Could you check a few things on this model? Use its own coordinates, in mm. A direction names the side the tool comes from. Round coordinates to 2 decimals unless told otherwise and drop trailing zeros. Loops run counter-clockwise (first coordinate to the right, second up) from the corner with the lowest first, then second, coordinate; pieces in that order, holes last. Notation, with made-up numbers: (-30, 3) -> (5, 3) arc R30 ccw to (5, 25) -> close; hole circle Ø11 at (9.5, 46.5). An arc over 180 degrees is marked (long way). Write each question's results on one line, items separated by ' | '. Start each with the question number.
1) Imagine slicing it at D-D, the plane z = -2.5. List the corners of the cut face in (x, y) for me.
2) Which directions (+Z, -Z, +X, -X, +Y, -Y) give clear straight access to the entire face, cutting with the end or side of a thin tool? Please do faces 4 (the flat face through (8.852, 21, 0)), 5 (the flat face through (4, 21.5, 2)), 6 (the flat face through (20, 8, 0)), 7 (the flat face through (-3, 15, 0)), 8 (the flat face through (-3, 15.8, 0)).
3) If I drill on probe 1 along Z at (x, y) = (21.5, 15.2); probe 2 along X at (y, z) = (9.25, -2.5); probe 3 along Y at (x, z) = (9.25, 0.5), over which ranges is the centre line in solid material (lowest first)?
4) Imagine slicing it at A-A, the plane z = 0. List the corners of the cut face in (x, y) for me, plus the area to 3 significant figures.
5) Imagine slicing it at C-C, the plane x = 4.15. List the corners of the cut face in (y, z) for me.
6) For P1, Ø4, axis at x = 22.5, z = -0.5, coming from the +Y side; P2, Ø1, axis at x = 12.5, z = 2, coming from the -Y side; P3, Ø3, axis at y = 11, z = 2.5, coming from the +X side; P4, Ø4, axis at y = 21, z = 2.5, coming from the -X side, each with a flat end and sliding along its axis, tell me the tip position at first contact or that it passes through.
7) We'd pull the mould along X, two halves only. Please class faces 1 (the cylindrical face through (5.935, 23.472, -0.234)), 2 (the cylindrical face through (22.5, 15.4, 0)), 3 (the flat face through (4, 25.5, 0)): pulls with the +X half, pulls with the -X half, needs draft (parallel to the pull), parting line crosses it, or undercut.
8) Imagine slicing it at B-B, the plane x = 21.5. List the corners of the cut face in (y, z) for me.
from build123d import *

# Parameters (mm, degrees)
EXTRUDE_1_DEPTH     = 4.15
SKETCH_2_W          = 27.3
SKETCH_2_H          = 0.8
EXTRUDE_2_DEPTH     = 8.3
CUT_EXTRUDE_1_REACH = 30.743
SKETCH_3_R          = 1
SKETCH_4_R          = 1.8
EXTRUDE_3_DEPTH     = 4


with BuildPart() as part:
    # Sketch 1 → Extrude 1 (new, symmetric)
    with BuildSketch(Plane.XY):
        Polygon((12.649672005, 19.5), (20, 17.950931016), (20, 0), (0, 0), (0, 16.33633198), (0, 21.5), (8.852277233, 21.5), (8.852277233, 19.5), align=None)
    extrude(amount=EXTRUDE_1_DEPTH, both=True)

    # Sketch 2 → Extrude 2 (add)
    with BuildSketch(Plane.XY.offset(4.15)):
        with Locations((10, 15.4)):
            Rectangle(SKETCH_2_W, SKETCH_2_H)
    extrude(amount=-EXTRUDE_2_DEPTH)

    # Sketch 3 → Cut-Extrude 1 (cut, up to next)
    with BuildSketch(Plane(origin=(0, 15.8, 0), x_dir=(1, 0, 0), z_dir=(0, 1, 0)), mode=Mode.PRIVATE) as cut_extrude_1_sk1:
        with Locations(Location((-1.5, 0, 0), (0, 0, 180))):
            Circle(SKETCH_3_R)
    cut_extrude_1_tool1 = extrude(cut_extrude_1_sk1.sketch, amount=-CUT_EXTRUDE_1_REACH, mode=Mode.PRIVATE) & part.part
    # Sketch 3 → Cut-Extrude 1 (cut, up to next)
    with BuildSketch(Plane(origin=(0, 15.8, 0), x_dir=(1, 0, 0), z_dir=(0, 1, 0)), mode=Mode.PRIVATE) as cut_extrude_1_sk2:
        with Locations(Location((21.5, 0, 0), (0, 0, 180))):
            Circle(SKETCH_3_R)
    cut_extrude_1_tool2 = extrude(cut_extrude_1_sk2.sketch, amount=-CUT_EXTRUDE_1_REACH, mode=Mode.PRIVATE) & part.part
    add(cut_extrude_1_tool1.solids().sort_by_distance((-1.5, 15.8, 0))[0], mode=Mode.SUBTRACT)
    add(cut_extrude_1_tool2.solids().sort_by_distance((21.5, 15.8, 0))[0], mode=Mode.SUBTRACT)

    # Sketch 4 → Extrude 3 (add)
    with BuildSketch(Plane(origin=(0, 21.5, 0), x_dir=(1, 0, 0), z_dir=(0, 1, 0))):
        with Locations(Location((4.15, 0, 0), (0, 0, 270))):
            Circle(SKETCH_4_R)
    extrude(amount=EXTRUDE_3_DEPTH)


solid = part.part
Checked values:
1) outline: (-3.65, 15) -> (0, 15) -> (0, 0) -> (20, 0) -> (20, 15) -> (23.65, 15) -> (23.65, 15.8) -> (20, 15.8) -> (20, 17.95) -> (12.65, 19.5) -> (8.85, 19.5) -> (8.85, 21.5) -> (0, 21.5) -> (0, 15.8) -> (-3.65, 15.8) -> close
2) face 4: +Z, -Z, +X, +Y | face 5: +Y | face 6: +Z, -Z, +X, -Y | face 7: +Z, -Z, -X, -Y | face 8: +Z, -Z, -X, +Y
3) probe 1: -4.15 to -1, 1 to 4.15 | probe 2: 0 to 20 | probe 3: 0 to 19.5
4) outline: (-3.65, 15) -> (-2.5, 15) -> (-2.5, 15.8) -> (-3.65, 15.8) -> close; (-0.5, 15) -> (0, 15) -> (0, 0) -> (20, 0) -> (20, 15) -> (20.5, 15) -> (20.5, 15.8) -> (20, 15.8) -> (20, 17.95) -> (12.65, 19.5) -> (8.85, 19.5) -> (8.85, 21.5) -> (5.95, 21.5) -> (5.95, 25.5) -> (2.35, 25.5) -> (2.35, 21.5) -> (0, 21.5) -> (0, 15.8) -> (-0.5, 15.8) -> close; (22.5, 15) -> (23.65, 15) -> (23.65, 15.8) -> (22.5, 15.8) -> close | area: 419 mm^2
5) outline: (0, -4.15) -> (21.5, -4.15) -> (21.5, -1.8) -> (25.5, -1.8) -> (25.5, 1.8) -> (21.5, 1.8) -> (21.5, 4.15) -> (0, 4.15) -> close
6) P1: y = 15.8 | P2: y = 0 | P3: x = 20 | P4: x = 0
7) face 1: parting line crosses it | face 2: undercut | face 3: needs draft
8) outline: (15, -4.15) -> (15.8, -4.15) -> (15.8, -1) -> (15, -1) -> close; (15, 1) -> (15.8, 1) -> (15.8, 4.15) -> (15, 4.15) -> close
